```python
from build123d import *

# Parameters (mm, degrees)
SKETCH1_W             = 61.48
SKETCH1_H             = 61.48
SKETCH1_R             = 2.2479
SKETCH1_R_2           = 19.812
BOSS_EXTRUDE1_DEPTH   = 5.08
FILLET1_R             = 2.54
BOSS_EXTRUDE2_DEPTH   = 5.08
SKETCH8_W             = 76.2
SKETCH8_H             = 76.2
SKETCH8_W_2           = 61.48
SKETCH8_H_2           = 61.48
BOSS_EXTRUDE3_DEPTH   = 5.08
F_8_CLEARANCE_HOLE1_D = 4.4958
FILLET2_R             = 2.54


with BuildPart() as part:
    # Sketch1 → Boss-Extrude1 (new body)
    with BuildSketch(Plane.XY):
        Rectangle(SKETCH1_W, SKETCH1_H)
        with Locations((-23.57, 23.57)):
            Circle(SKETCH1_R, mode=Mode.SUBTRACT)
        with Locations((-23.57, -23.57)):
            Circle(SKETCH1_R, mode=Mode.SUBTRACT)
        with Locations((23.57, -23.57)):
            Circle(SKETCH1_R, mode=Mode.SUBTRACT)
        Circle(SKETCH1_R_2, mode=Mode.SUBTRACT)
        with Locations((23.57, 23.57)):
            Circle(SKETCH1_R, mode=Mode.SUBTRACT)
    extrude(amount=BOSS_EXTRUDE1_DEPTH)

    # Fillet1
    fillet1_edges = [part.edges().sort_by_distance(p)[0] for p in [
        (-30.74, 30.74, 2.54),
        (30.74, 30.74, 2.54),
        (30.74, -30.74, 2.54),
        (-30.74, -30.74, 2.54),
    ]]
    fillet(fillet1_edges, radius=FILLET1_R)

    # Sketch7 → Boss-Extrude2 (add, through all)
    with BuildSketch(Plane(origin=(0, 0, 0), x_dir=(-1, 0, 0), z_dir=(0, 0, -1))):
        with BuildLine():
            Line((-27.259871939, 36.240128061), (-21.759743879, 30.74))
            Line((-21.759743879, 30.74), (-30.74, 21.759743879))
            Line((-30.74, 21.759743879), (-36.240128061, 27.259871939))
            ThreePointArc((-36.240128061, 27.259871939), (-36.240128061, 36.240128061), (-27.259871939, 36.240128061))
        make_face()
        with BuildLine():
            Line((30.74, 21.759743879), (36.240128061, 27.259871939))
            ThreePointArc((36.240128061, 27.259871939), (36.240128061, 36.240128061), (27.259871939, 36.240128061))
            Line((27.259871939, 36.240128061), (21.759743879, 30.74))
            Line((21.759743879, 30.74), (30.74, 21.759743879))
        make_face()
        with BuildLine():
            Line((27.259871939, -36.240128061), (21.759743879, -30.74))
            Line((21.759743879, -30.74), (30.74, -21.759743879))
            Line((30.74, -21.759743879), (36.240128061, -27.259871939))
            ThreePointArc((36.240128061, -27.259871939), (36.240128061, -36.240128061), (27.259871939, -36.240128061))
        make_face()
        with BuildLine():
            Line((-30.74, -21.759743879), (-36.240128061, -27.259871939))
            ThreePointArc((-36.240128061, -27.259871939), (-36.240128061, -36.240128061), (-27.259871939, -36.240128061))
            Line((-27.259871939, -36.240128061), (-21.759743879, -30.74))
            Line((-21.759743879, -30.74), (-30.74, -21.759743879))
        make_face()
    extrude(amount=-BOSS_EXTRUDE2_DEPTH)

    # Sketch8 → Boss-Extrude3 (add, through all)
    with BuildSketch(Plane(origin=(0, 0, 0), x_dir=(-1, 0, 0), z_dir=(0, 0, -1))):
        Rectangle(SKETCH8_W, SKETCH8_H)
        Rectangle(SKETCH8_W_2, SKETCH8_H_2, mode=Mode.SUBTRACT)
    extrude(amount=-BOSS_EXTRUDE3_DEPTH)

    # #8 Clearance Hole1 (through all)
    with Locations(Plane(origin=(0, 0, 0), x_dir=(-1, 0, 0), z_dir=(0, 0, -1))):
        with Locations((31.75, 31.75), (0, 0), (31.75, -31.75), (-31.75, -31.75), (-31.75, 31.75)):
            Hole(F_8_CLEARANCE_HOLE1_D / 2)

    # Fillet2
    fillet2_edges = [part.edges().sort_by_distance(p)[0] for p in [
        (-38.1, 38.1, 2.54),
        (-38.1, -38.1, 2.54),
        (38.1, -38.1, 2.54),
        (38.1, 38.1, 2.54),
    ]]
    fillet(fillet2_edges, radius=FILLET2_R)


solid = part.part
```
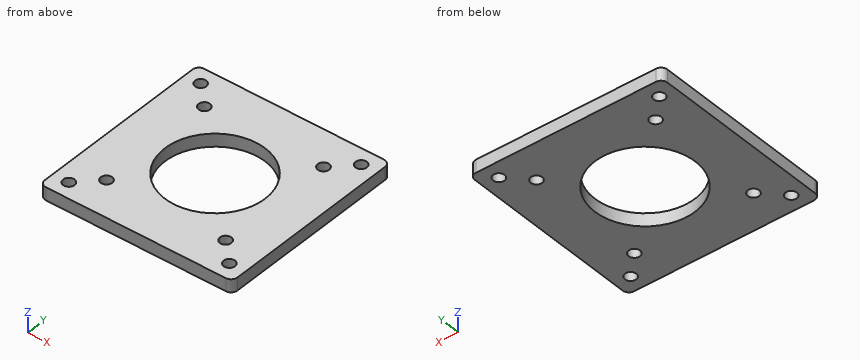
Could you check a few things on this model? Use its own coordinates, in mm. Round coordinates to 2 decimals unless told otherwise and drop trailing zeros. Write each loop counter-clockwise with the first axis right and the second up, starting at its lowest first coordinate (ties: lowest second). Pieces come first, ordered by that corner, then holes. Notation, with made-up numbers: M -29.75,72 L 3.25,72 A6 ccw 3.25,76 Z; hole C 1,62 d7. An arc over 180 degrees is marked long. Answer in a Markdown table with one row per item. Add a question column.
Q1. Imagine slicing it at C-C (x = 0). Please give me the cut outline in (y, z), then the cut area to 3 significant figures.
Q2. Imagine slicing it at A-A (x = 23.57). Please give me the cut outline in (y, z), then the cut area to 3 significant figures.
Q3. If I drill on line 1 (X direction, y = 32, z = 4.15); line 2 (Y direction, x = -23.57, z = 3.8), over which ranges is the centre line in solid material (lowest first)? Write a range as from..to.
Values:
| question | item | result |
|---|---|---|
| 1 | outline | M -38.1,0 L -19.81,0 L -19.81,5.08 L -38.1,5.08 Z; M 19.81,0 L 38.1,0 L 38.1,5.08 L 19.81,5.08 Z |
| 1 | area | 186 mm^2 |
| 2 | outline | M -38.1,0 L -25.82,0 L -25.82,5.08 L -38.1,5.08 Z; M -21.32,0 L 21.32,0 L 21.32,5.08 L -21.32,5.08 Z; M 25.82,0 L 38.1,0 L 38.1,5.08 L 25.82,5.08 Z |
| 2 | area | 341 mm^2 |
| 3 | line 1 | -38.1..-33.98, -29.52..29.52, 33.98..38.1 |
| 3 | line 2 | -38.1..-25.82, -21.32..21.32, 25.82..38.1 |
